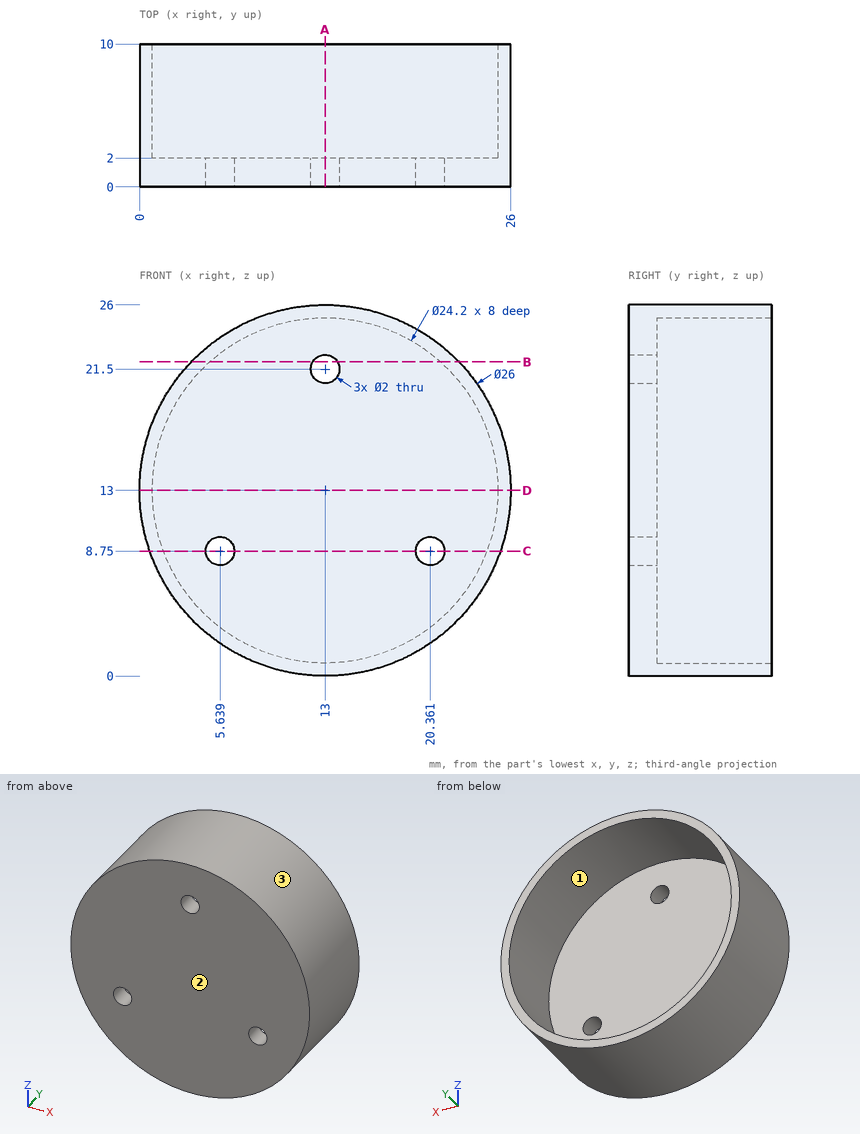
Verification items for this drawing (mm, ordinates from the low corner). Coordinates: 2 decimals unless noted, no trailing zeros. Loops run counter-clockwise (first coordinate to the right, second up) from the corner with the lowest first, then second, coordinate; pieces in that order, holes last. Notation, with made-up numbers: (58, 54) - (106, 54) arc R12 ccw to (106, 70) - close; hole circle Ø1 at (44, -15). An arc over 180 degrees is marked (long way). One line per item, written item: value. Start each with the question number.
(1) Cross-section at D-D on z = 13. Enter the section's corners in (x, y), plus the area to 3 significant figures.
(2) Depth check by flat-ended pin: P1, Ø12, axis at x = 16.5, z = 15.5, coming from the +Y side; P2, Ø1.5, axis at y = 6, z = 16.5, coming from the +X side; P3, Ø6, axis at x = 2.5, y = 3.5, coming from the +Z side. Enter the tip coordinate at first touch or a pass-through.
(3) Cross-section at C-C on z = 8.75. Enter the section's corners in (x, y).
(4) Cross-section at B-B on z = 22. Enter the section's corners in (x, y).
(5) Mould release check, pull along X, two halves, no side actions. Record for the marked faces 1, 2 and 3: released by +X, released by -X, zero draft, split by the parting line, or undercut.
(6) Material ranges on line 1 (X direction, y = 7, z = 13); line 2 (Y direction, x = 23.5, z = 14.5), recorded low to high. Write a range as [from, to].
(7) Cross-section at A-A on x = 13. Enter the section's corners in (y, z).
Results below:
1. outline: (0, 0) - (26, 0) - (26, 10) - (25.1, 10) - (25.1, 2) - (0.9, 2) - (0.9, 10) - (0, 10) - close
1. area: 66.4 mm2
2. P1: stops at y = 2
2. P2: stops at x = 25.71
2. P3: stops at z = 23.62
3. outline: (0.71, 0) - (4.64, 0) - (4.64, 2) - (1.67, 2) - (1.67, 10) - (0.71, 10) - close; (6.64, 0) - (19.36, 0) - (19.36, 2) - (6.64, 2) - close; (21.36, 0) - (25.29, 0) - (25.29, 10) - (24.33, 10) - (24.33, 2) - (21.36, 2) - close
4. outline: (3.62, 0) - (12.13, 0) - (12.13, 2) - (4.91, 2) - (4.91, 10) - (3.62, 10) - close; (13.87, 0) - (22.38, 0) - (22.38, 10) - (21.09, 10) - (21.09, 2) - (13.87, 2) - close
5. face 1: undercut
5. face 2: zero draft
5. face 3: split by the parting line
6. line 1: x = [0, 0.9], [25.1, 26]
6. line 2: y = [0, 2]
7. outline: (0, 0) - (10, 0) - (10, 0.9) - (2, 0.9) - (2, 20.5) - (0, 20.5) - close; (0, 22.5) - (2, 22.5) - (2, 25.1) - (10, 25.1) - (10, 26) - (0, 26) - close
